Source: CAD feature listing. Evaluate the final solid. Frame: model axes, mm. A direction names the side the tool comes from. Round coordinates to 2 decimals unless told otherwise and drop trailing zeros. Write each loop counter-clockwise with the first axis right and the second up, starting at its lowest first coordinate (ties: lowest second). Pieces come first, ordered by that corner, then holes. Notation, with made-up numbers: (47.25, -31) - (62.25, -31) arc R17 ccw to (62.25, -5) - close; hole circle Ø9 at (3, 67.25). An arc over 180 degrees is marked (long way). Write item = value, one per line. Start each with the question number.
Autodesk Inventor part; units mm, degrees
ref_plane "YZ Plane" through (0, 0, 0) normal (1, 0, 0) x (0, 1, 0)
ref_plane "XZ Plane" through (0, 0, 0) normal (0, 1, 0) x (-1, 0, 0)
ref_plane "XY Plane" through (0, 0, 0) normal (0, 0, 1) x (1, 0, 0)
ref_plane "Work Plane1" through (0, 0, 2.5) normal (0, 0, 1) x (1, 0, 0)
sketch "Sketch1" plane through (0, 0, 2.5) normal (0, 0, 1) x (1, 0, 0)
  circle A0 centre (0, 0) radius 9.75
  circle A1 centre (0, 0) radius 17.5
  line L0 (0, 0) -> (0, 47) construction
  line L1 (40, 47) -> (-40, 47)
  line L2 (-40, 47) -> (-15.996, -7.0977)
  line L3 (40, 47) -> (15.996, -7.0977)
  line L4 (-25.7319, 39.5) -> (25.7319, 39.5)
  line L5 (25.7319, 39.5) -> (13.2683, 11.4107)
  line L6 (-13.2683, 11.4107) -> (-25.7319, 39.5)
  dimension "d0" = 19.5
  dimension "d1" = 35
  dimension "d2" = 47
  dimension "d3" = 80
  dimension "d4" = 7.5
  dimension "d6" = 10
  dimension "d7" = 10
extrude "Extrusion1" add sketch "Sketch1" along normal blind 10 contours A1 | A1 L5 L4 L6 L2 L1 L3
sketch "Sketch2" plane through (-40, 47, 2.5) normal (0, 1, 0) x (1, 0, 0)
  line L0 (0, 0) -> (0, -10) construction
  line L1 (0, -5) -> (80, -5) construction
  line L2 (80, 0) -> (80, -10) construction
  circle A0 centre (15, -5) radius 1.35
  circle A1 centre (25, -5) radius 1.35
  line L3 (40, -5) -> (40, 0) construction
  line L4 (24.004, 0) -> (55.996, 0) construction
  circle A2 centre (65, -5) radius 1.35
  circle A3 centre (55, -5) radius 1.35
  circle A4 centre (40, -5) radius 3.5
  point P0 (40, 2.5)
  dimension "d10" = 2.7
  dimension "d11" = 15
  dimension "d14" = 10
  dimension "d19" = 7
extrude "Extrusion2" cut sketch "Sketch2" against normal up to surface (7.5 mm away)
ref_plane "Work Plane2" through (-40, 17.5, 2.5) normal (0, 1, 0) x (1, 0, 0)
sketch "Sketch3" plane through (-40, 17.5, 2.5) normal (0, 1, 0) x (1, 0, 0)
  circle A0 centre (40, -5) radius 3.5
  point P0 (40, 2.5)
extrude "Extrusion3" cut sketch "Sketch3" against normal blind 4
fillet "Fillet1" radius 1 3 edges at (2.669, 17.2953, 9.7641) (-3.4999, 17.1465, 7.4721) (2.6638, 17.2961, 5.2297)
properties part number "LowerWheelBracket"
(1) Contact query for flat-ended pins moving along their axis: P1, Ø5, axis at y = 3.5, z = 6, coming from the -X side; P2, Ø3, axis at y = 7.5, z = 5, coming from the -X side; P3, Ø17.5, axis at x = 0, y = 0, coming from the +Z side; P4, Ø4.5, axis at x = 15, z = 7.5, coming from the -Y side. Output: stop coordinate, or through.
(2) Section B-B (y = 35.5). Return the cut outline in (x, z), plus the area to 3 significant figures.
(3) Section D-D (x = 32.5). Return the cut outline in (y, z), plus the area to 3 significant figures.
(4) Reachability of faces 1 (the cylindrical face through (0.283, -17.498, 7.43)), 2 (the flat face through (-19.413, 25.259, 7.43)), 3 (the cylindrical face through (-15.176, 43.302, 6.161)) from +Z, -Z, +X, -X, +Y, -Y: full face, straight path, thin tool, end or side. Return the list, or none.
(5) Ray query, L1, parallel to Z at x = 15, y = 42; L2, parallel to Y at x = -4, z = 3.75; L3, parallel to X at y = 43.75, z = 7.5. Return the intervals inside material, ascending. Write a range as from..to.
(6) Section A-A (x = -11.5). Return the cut outline in (y, z).
(7) Section C-C (x = 0). Count the separate pieces of the cut face and the enclosed holes in it, plus the area to 3 significant figures.
(8) Pull-direction query (Z, two-part tool) for faces 4 (the flat face through (-1, 15, 2.5)), 5 (the cylindrical face through (-23.712, 43.302, 7.094)), 6 (the flat face through (-1, 15, 12.5)), 7 (the flat face through (-28.166, 20.33, 7.43)); classes: +Z half, -Z half, draft (parallel to the pull), parting line (faces both ways), or undercut.
Solution:
q1.P1 = -21.81
q1.P2 = -23.14
q1.P3 = through
q1.P4 = -11.99
q2.outline = (-34.9, 2.5) - (-23.96, 2.5) - (-23.96, 12.5) - (-34.9, 12.5) - close; (23.96, 2.5) - (34.9, 2.5) - (34.9, 12.5) - (23.96, 12.5) - close
q2.area = 219 mm^2
q3.outline = (30.1, 2.5) - (47, 2.5) - (47, 12.5) - (30.1, 12.5) - close
q3.area = 169 mm^2
q4.face_1 = +Z, -Z, -Y
q4.face_2 = +Z, -Z
q4.face_3 = +Y
q5.L1 = 2.5..6.15, 8.85..12.5
q5.L2 = -17.04..-8.89, 8.89..17.04, 39.5..47
q5.L3 = -38.56..-26.35, -23.65..-16.35, -13.65..-3.5, 3.5..13.65, 16.35..23.65, 26.35..38.56
q6.outline = (-13.19, 2.5) - (13.19, 2.5) - (13.19, 12.5) - (-13.19, 12.5) - close; (39.5, 2.5) - (47, 2.5) - (47, 12.5) - (39.5, 12.5) - close
q7.separate_pieces = 4
q7.enclosed_holes = 0
q7.area = 149 mm^2
q8.face_4 = -Z half
q8.face_5 = undercut
q8.face_6 = +Z half
q8.face_7 = draft
